Autodesk Inventor part; units mm, degrees
ref_plane "YZ Plane" through (0, 0, 0) normal (1, 0, 0) x (0, 1, 0)
ref_plane "XZ Plane" through (0, 0, 0) normal (0, 1, 0) x (-1, 0, 0)
ref_plane "XY Plane" through (0, 0, 0) normal (0, 0, 1) x (1, 0, 0)
sketch "Sketch1" plane through (0, 0, 0) normal (0, 1, 0) x (-1, 0, 0)
  line L0 (0, 0) -> (0, -30)
  circle A0 centre (0, 5) radius 5
  circle A1 centre (0, -35) radius 5
  line L1 (-5, 5) -> (-14, 5) construction
  line L2 (0, 10) -> (0, 15) construction
  line L3 (0, 10) -> (-14, 10) construction
  line L4 (5, 5) -> (10, 5) construction
  line L5 (-14, 5) -> (-11.1, 5) construction
  line L6 (0, 0) -> (-14, 0) construction
  line L7 (-11.1, 0) -> (-11.1, 1) construction
  line L8 (5, -35) -> (10, -35) construction
  line L9 (0, -40) -> (0, -45) construction
  line L10 (-5, -35) -> (-14, -35) construction
  line L11 (0, -40) -> (-14, -40) construction
  line L12 (0, -30) -> (-14, -30) construction
  line L13 (-11.1, -30) -> (-11.1, -31) construction
  line L14 (-14, 10) -> (0, 15)
  line L15 (0, 15) -> (10, 18.5714)
  line L16 (-14, -40) -> (0, -45)
  line L17 (0, -45) -> (10, -48.5714)
  line L18 (10, -48.5714) -> (10, 18.5714)
  line L19 (-14, 10) -> (-14, 5)
  line L20 (-11.1, 1) -> (-11.1, -31)
  line L21 (-14, -40) -> (-14, -35)
  line L22 (-14, 10) -> (-14, 3.9) construction
  line L23 (-14, -40) -> (-14, -33.9) construction
  line L24 (-11.1, 1) -> (-14, 4.45)
  line L25 (-11.1, -31) -> (-14, -34.45)
  line L26 (-14, 4.45) -> (-14, 5)
  line L27 (-14, -34.45) -> (-14, -35)
  dimension "d0" = 30
  dimension "d3" = 9
  dimension "d4" = 5
  dimension "d5" = 5
  dimension "d6" = 2.9
  dimension "d7" = 1
  dimension "d8" = 5
  dimension "d9" = 1
  dimension "d10" = 6.1
  dimension "d11" = 6.1
extrude "Extrusion3" add sketch "Sketch1" along normal blind 3
sketch "Sketch4" plane through (0, 3, 0) normal (0, 1, 0) x (1, 0, 0)
  circle A0 centre (0, 35) radius 5
  circle A1 centre (0, -5) radius 5
  point P0 (0, 0)
sketch "Sketch5" plane through (0, 3, 0) normal (0, 1, 0) x (1, 0, 0)
  point P0 (0, 0)
extrude "Extrusion4" add sketch "Sketch4" along normal blind 5
sketch "Sketch6" plane through (0, 8, 5) normal (0, 1, 0) x (1, 0, 0)
  circle A0 centre (0, 0) radius 5.5
  circle A1 centre (0, 40) radius 5
  circle A2 centre (0, 40) radius 5.5
  point P0 (0, 5)
  dimension "d20" = 11
  dimension "d21" = 11
extrude "Extrusion5" add sketch "Sketch6" along normal blind 3 contours A0 | A1 | A2
fillet "Fillet1" radius 2 2 edges at (-5.5, 11, 5) (-5.5, 11, -35)
sketch "Sketch7" plane through (0, 11, 5) normal (0, 1, 0) x (1, 0, 0)
  circle A0 centre (0, 0) radius 3.5
  circle A1 centre (0, 40) radius 3.5
  circle A2 centre (0, 0) radius 5.5
  line L0 (-5.5, 0) -> (-5.5, 1)
  line L1 (-5.5, 1) -> (5.5, 1)
  line L2 (5.5, 1) -> (5.5, -1)
  line L3 (5.5, -1) -> (-5.5, -1)
  line L4 (-5.5, -1) -> (-5.5, 0)
  line L5 (-5.5, 40) -> (-5.5, 41)
  line L6 (-5.5, 41) -> (5.5, 41)
  line L7 (5.5, 41) -> (5.5, 39)
  line L8 (5.5, 39) -> (-5.5, 39.0974)
  line L9 (-5.5, 39.0974) -> (-5.5, 40)
  circle A3 centre (0, 40) radius 5.5
  point P0 (0, 5)
  dimension "d25" = 1
  dimension "d26" = 2
  dimension "d27" = 1
  dimension "d28" = 2
extrude "Extrusion6" cut sketch "Sketch7" against normal blind 7 contours A0 L3 L1 | A0 L1 A2 L3 | A0 L3 A2 L1 | L1 L2 A2 | A2 L2 L3 | A2 L0 L1 | L3 L4 A2 | A1 L8 L6 | A1 L6 A3 L8 | A1 L8 A3 L6 | L6 L7 A3 | A3 L7 L8 | A3 L5 L6 | L8 L9 A3
fillet "Fillet2" radius 0.6 4 edges at (0, 4, 6) (0, 4, 4) (-0.0084, 4, -34.0488) (0, 4, -36)
sketch "Sketch8" plane through (0, 0, 0) normal (0, -1, 0) x (1, 0, 0)
  circle A0 centre (0, 5) radius 5
  circle A1 centre (0, -35) radius 5
  point P0 (0, 0)
extrude "Extrusion7" add sketch "Sketch8" against normal blind 3
sketch "Sketch9" plane through (0, 3, 0) normal (0, 1, 0) x (1, 0, 0)
  circle A0 centre (0, 35) radius 5
  circle A1 centre (0, -5) radius 5
  line L0 (14, -10) -> (14, -4.45)
  line L1 (14, -4.45) -> (11.1, -1)
  line L2 (11.1, -1) -> (11.1, 31)
  line L3 (11.1, 31) -> (14, 34.45)
  line L4 (14, 34.45) -> (14, 40)
  line L5 (14, 40) -> (-10, 48.5714)
  line L6 (-10, 48.5714) -> (-10, -18.5714)
  line L7 (-10, -18.5714) -> (14, -10)
  line L8 (14, -10) -> (16, -10)
  line L9 (16, -10) -> (16, 40)
  line L10 (16, 40) -> (14, 40)
  point P0 (0, 0)
  dimension "d34" = 2
extrude "Extrusion8" add sketch "Sketch9" along normal blind 105 contours L0 L1 L2 L3 L4 L10 L9 L8
sketch "Sketch10" plane through (0, 0, 0) normal (0, -1, 0) x (1, 0, 0)
  line L0 (14, 4.45) -> (14, 10)
  line L1 (14, 10) -> (-10, 18.5714)
  line L2 (-10, 18.5714) -> (-10, -48.5714)
  line L3 (-10, -48.5714) -> (14, -40)
  line L4 (14, -40) -> (14, -34.45)
  line L5 (14, -34.45) -> (11.1, -31)
  line L6 (11.1, -31) -> (11.1, 1)
  line L7 (11.1, 1) -> (14, 4.45)
  line L8 (14, 10) -> (16, 10)
  line L9 (14, 10) -> (14, 4.45)
  line L10 (14, 4.45) -> (11.1, 1)
  line L11 (11.1, 1) -> (11.1, -31)
  line L12 (11.1, -31) -> (14, -34.45)
  line L13 (14, -34.45) -> (14, -40)
  line L14 (16, -40) -> (14, -40)
  line L15 (16, 10) -> (16, -40)
  point P0 (0, 0)
extrude "Extrusion9" add sketch "Sketch10" against normal blind 3 contours L0 L8 L15 L14 L4 L5 L6 L7
fillet "Fillet3" radius 0.8 4 edges at (11.1, 55.5, 1) (14, 55.5, 4.45) (14, 55.5, -34.45) (11.1, 55.5, -31)
sketch "Sketch11" plane through (0, 3, 0) normal (0, 1, 0) x (1, 0, 0)
  arc A0 (13.8124, 34.2268) -> (14, 34.7416) centre (13.2, 34.7416) ccw
  line L0 (14, 34.7416) -> (14, 40)
  line L1 (14, 40) -> (-10, 48.5714)
  line L2 (-10, 48.5714) -> (-10, -18.5714)
  line L3 (-10, -18.5714) -> (14, -10)
  line L4 (14, -10) -> (14, -4.7416)
  arc A1 (14, -4.7416) -> (13.8124, -4.2268) centre (13.2, -4.7416) ccw
  line L5 (13.8124, -4.2268) -> (11.2876, -1.2232)
  arc A2 (11.1, -0.7084) -> (11.2876, -1.2232) centre (11.9, -0.7084) ccw
  line L6 (11.1, -0.7084) -> (11.1, 30.7084)
  arc A3 (11.2876, 31.2232) -> (11.1, 30.7084) centre (11.9, 30.7084) ccw
  line L7 (11.2876, 31.2232) -> (13.8124, 34.2268)
  circle A4 centre (0, -5) radius 5
  circle A5 centre (0, 35) radius 5
  line L8 (-10, 48.5714) -> (-10, -18.5714)
  line L9 (-10, 48.5714) -> (-10, 52.4265)
  line L10 (11.1, 40) -> (23.5531, 40)
  line L11 (16, 40) -> (14, 40)
  line L12 (16, 40) -> (-10, 49.2857)
  line L13 (14, -10) -> (19.1534, -10)
  line L14 (-10, -18.5714) -> (14, -10)
  line L15 (-10, -18.5714) -> (-10, -22.2627)
  line L16 (16, -10) -> (16, 40)
  line L17 (16, -10) -> (-10, -19.2857)
  point P0 (0, 0)
extrude "Extrusion10" add sketch "Sketch11" along normal blind 5 contours L1 L9 L12 L10 | L3 L13 L17 L15
sketch "Sketch12" plane through (0, 0, 0) normal (0, -1, 0) x (1, 0, 0)
  line L0 (14, -40) -> (16, -40)
  line L1 (14, -40) -> (-10, -48.5714)
  line L2 (-10, -49.2857) -> (-10, -48.5714)
  line L3 (16, -40) -> (-10, -49.2857)
  line L4 (-10, 18.5714) -> (-10, 19.2857)
  line L5 (-10, 18.5714) -> (14, 10)
  line L6 (16, 10) -> (14, 10)
  line L7 (-10, 19.2857) -> (16, 10)
  point P0 (0, 0)
extrude "Extrusion11" add sketch "Sketch12" against normal blind 3
properties part number "SOPORTE"
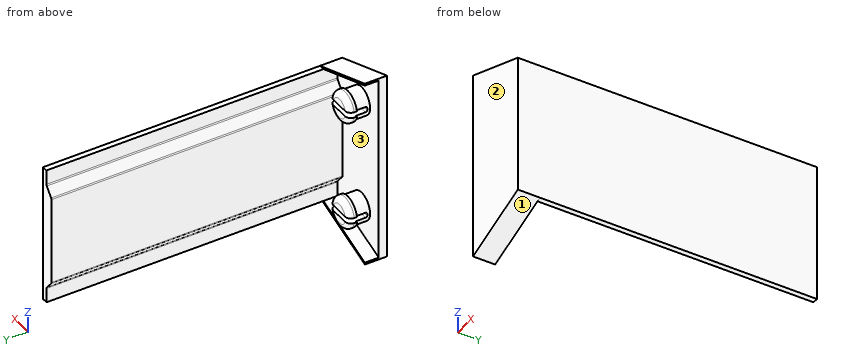
The model under review builds one solid part; all positions refer to its coordinate system, in mm. Face numbers are marked on the shaded views. Coordinates: 2 decimals unless noted, no trailing zeros. Write each loop counter-clockwise with the first axis right and the second up, starting at its lowest first coordinate (ties: lowest second). Pieces come first, ordered by that corner, then holes. Notation, with made-up numbers: (-36.75, 15) - (-30.75, 15) arc R27 ccw to (-30.75, 48) - close; hole circle Ø11 at (81, 81). An arc over 180 degrees is marked (long way). Answer in a Markdown table with one row per item. Add a question column.
Q1. Clearance check with flat-ended pins moving along their axes: pin 1 (15.5 mm diameter, centred on y = 80.5, z = -18, fed in from -X); pin 2 (2 mm diameter, centred on x = -0.5, z = 3, fed in from +Y); pin 3 (7.5 mm diameter, centred on x = -1.5, z = 14.5, fed in from +Y); pin 4 (5 mm diameter, centred on x = 6.5, y = 83.5, fed in from -Z). State where each tip first meets the part, or that it passes through.
Q2. Draft analysis for pull direction Z (two halves, no side actions). For the marked faces 1, 2 and 3, state which applies: +Z half, -Z half, draft (parallel to the pull), parting line (faces both ways), or undercut.
Q3. Consider section B-B on z = -18. Give the boundary of the cut face in (x, y), then the cut area to 4 significant figures.
Q4. To check wall thickness, follow line 1 along X through (y, z) = (63, -35); line 2 along Y through (x, z) = (-7.5, -18); line 3 along X through (y, z) = (31.5, -10.5). State the ranges of each line that lie inside material, in increasing order. Write a range as from..to.
Q5. Consider section C-C on x = 7.5. Give the boundary of the cut face in (y, z), then the cut area to 3 significant figures.
Q6. Consider section A-A on y = 86. Give the boundary of the cut face in (x, z), then the cut area to 3 significant figures.
Q7. Consider section D-D on z = 14. Give the boundary of the cut face in (x, y).
Answers below:
| question | item | result |
|---|---|---|
| 1 | pin 1 | x = 11.1 |
| 1 | pin 2 | y = 11 |
| 1 | pin 3 | y = 8 |
| 1 | pin 4 | through |
| 2 | face 1 | -Z half |
| 2 | face 2 | draft |
| 2 | face 3 | undercut |
| 3 | outline | (-10, 0) - (16, 0) - (16, 108) - (11.1, 108) - (11.1, 3) - (-10, 3) - close |
| 3 | area | 592.5 mm² |
| 4 | line 1 | 14..16 |
| 4 | line 2 | 0..3 |
| 4 | line 3 | 11.1..16 |
| 5 | outline | (0, -43.04) - (8, -43.04) - (8, -42.32) - (3, -42.32) - (3, 12.32) - (8, 12.32) - (8, 13.04) - (0, 13.04) - close |
| 5 | area | 175 mm² |
| 6 | outline | (11.1, -30.71) arc R0.8 ccw to (11.29, -31.22) - (13.81, -34.23) arc R0.8 cw to (14, -34.74) - (14, -40) - (16, -40) - (16, 10) - (14, 10) - (14, 4.74) arc R0.8 cw to (13.81, 4.23) - (11.29, 1.22) arc R0.8 ccw to (11.1, 0.71) - close |
| 6 | area | 203 mm² |
| 7 | outline | (-10, 0) - (4.8, 0) - (4.8, 8) - (2.8, 8) - (2.8, 3) - (-10, 3) - close |
